Here's how the part is built. I have some questions about the finished solid (model axes, mm). A direction names the side the tool comes from. Coordinates: 2 decimals unless noted, no trailing zeros. Order: outer loops, then holes, each group sorted by start corner. A loop starts at its lowest first (then second) coordinate and runs counter-clockwise, first axis right, second up. Notation, with made-up numbers: M 87,-11.75 L 145,-11.75 A19 cw 145,-1.75 Z; hole C 70.25,70.25 d2. An arc over 180 degrees is marked long. Answer as CSV lines item,"result". Start each with the question number.
Autodesk Inventor part; units mm, degrees
ref_plane "YZ Plane" through (0, 0, 0) normal (1, 0, 0) x (0, 1, 0)
ref_plane "XZ Plane" through (0, 0, 0) normal (0, 1, 0) x (-1, 0, 0)
ref_plane "XY Plane" through (0, 0, 0) normal (0, 0, 1) x (1, 0, 0)
sketch "Esquisse1" plane through (0, 0, 0) normal (0, 1, 0) x (-1, 0, 0)
  line L0 (2.8537, 2.5756) -> (-12.1463, 2.5756)
  line L1 (-12.1463, 2.5756) -> (-12.1463, -7.4244)
  line L2 (-12.1463, -7.4244) -> (2.8537, -7.4244)
  line L3 (2.8537, -7.4244) -> (2.8537, 2.5756)
  point P0 (0, 0)
  dimension "d0" = 10
  dimension "d1" = 15
extrude "Extrusion1" add sketch "Esquisse1" along normal blind 3
sketch "Esquisse2" plane through (0, 3, 0) normal (0, 1, 0) x (1, 0, 0)
  line L0 (-2.8537, 7.4244) -> (-2.8537, -2.5756)
  line L1 (12.1463, 7.4244) -> (-2.8537, 7.4244)
  line L2 (-2.8537, -2.5756) -> (0.1463, -2.5756)
  line L3 (0.1463, -2.5756) -> (0.1463, 7.4244)
  line L4 (0.1463, 7.4244) -> (-2.8537, 7.4244)
  line L5 (-2.8537, 7.4244) -> (-2.8537, -2.5756)
  point P0 (0, 0)
  dimension "d4" = 3
extrude "Extrusion2" add sketch "Esquisse2" along normal blind 40
sketch "Esquisse3" plane through (0, 3, 0) normal (0, 1, 0) x (1, 0, 0)
  circle A0 centre (3.1463, 2.4244) radius 1.5
  circle A1 centre (9.1463, 2.4244) radius 1.5
  line L0 (12.1463, -2.5756) -> (12.1463, 7.4244)
  line L1 (0.1463, -2.5756) -> (12.1463, -2.5756)
  line L2 (0.1463, -2.5756) -> (0.1463, 7.4244)
  point P0 (0, 0)
  dimension "d7" = 3
  dimension "d8" = 3
  dimension "d9" = 3
  dimension "d10" = 5
  dimension "d11" = 5
  dimension "d12" = 3
extrude "Extrusion3" cut sketch "Esquisse3" against normal through all
sketch "Esquisse4" plane through (0, 3, 0) normal (0, 1, 0) x (1, 0, 0)
  line L0 (0.1463, -2.5756) -> (12.1463, -2.5756)
  line L1 (0.1463, -2.5756) -> (5.1463, -2.5756)
  line L2 (5.1463, -2.5756) -> (5.1463, -1.5756)
  line L3 (5.1463, -1.5756) -> (0.1463, -1.5756)
  line L4 (0.1463, -1.5756) -> (0.1463, -2.5756)
  line L5 (12.1463, 7.4244) -> (0.1463, 7.4244)
  line L6 (0.1463, 7.4244) -> (5.1463, 7.4244)
  line L7 (5.1463, 7.4244) -> (5.1463, 6.4244)
  line L8 (5.1463, 6.4244) -> (0.1463, 6.4244)
  line L9 (0.1463, 6.4244) -> (0.1463, 7.4244)
  point P0 (0, 0)
  dimension "d15" = 1
  dimension "d16" = 1
  dimension "d17" = 5
extrude "Extrusion4" add sketch "Esquisse4" along normal blind 5
chamfer "Chanfrein1" distance 5 angle 45 1 edges at (5.1463, 8, 2.0756)
chamfer "Chanfrein2" distance 5 angle 45 1 edges at (5.1463, 8, -6.9244)
sketch "Esquisse5" plane through (0.1463, 43, 2.5756) normal (1, 0, 0) x (0, 0, -1)
  circle A0 centre (5, -3) radius 1.5
  line L0 (0, -35) -> (0, 0)
  line L1 (0, 0) -> (10, 0)
  point P0 (2.5756, -43)
  dimension "d26" = 3
  dimension "d27" = 5
  dimension "d28" = 3
extrude "Extrusion5" cut sketch "Esquisse5" against normal through all
properties part number "equerre-bras"
1) Suppose I cut it at B-B on z = -2. Please give me the cut outline in (x, y) (3 decimals).
2) Suppose I cut it at A-A on y = 40. Please give me the cut outline in (x, z), plus the area to 3 significant figures.
3) I need wall thicknesses on line 1 (X direction, y = 36, z = 0); line 2 (Y direction, x = 3.75, z = -5); line 3 (Y direction, x = -2, z = -3). Which ranges of each line are inside material? Lowest first, please. Write a range as [from, to].
4) Which directions (+Z, -Z, +X, -X, +Y, -Y) give clear straight access to the entire face, cutting with the end or side of a thin tool? Please do faces 4 (the face through (-1, 43, -2)), 5 (the face through (2, 5, 1.576)).
5) Suppose I cut it at C-C on x = -1.75. Please give me the cut outline in (y, z), plus the area to 3 significant figures.
6) If we mould it in two halves opening along X, with no side actions, what happens to faces 1 (the face through (-1.333, 38.536, -2.099)), 2 (the face through (12.146, 1, -2)), 3 (the face through (3.95, 1.52, -3.69))? For each: released by +X, released by -X, zero draft, split by the parting line, or undercut.
7) Will these pins go through, and if not, where does the flat tip stop? pin 1 Ø3 at (x, z) = (6.5, -4) entering from +Y; pin 2 Ø5 at (y, z) = (40, -2.42) entering from +X; pin 3 Ø8 at (x, y) = (8, 9) entering from +Z.
8) Suppose I cut it at D-D on x = 3.5. Please give me the cut outline in (y, z), plus the area to 3 significant figures.
Output:
1,outline,"M -2.854,0 L 1.708,0 L 1.708,3 L 0.146,3 L 0.146,38.561 L -2.854,38.561 Z; M -2.854,41.439 L 0.146,41.439 L 0.146,43 L -2.854,43 Z; M 4.585,0 L 7.708,0 L 7.708,3 L 4.585,3 Z; M 10.585,0 L 12.146,0 L 12.146,3 L 10.585,3 Z"
2,outline,"M -2.85,-7.42 L 0.15,-7.42 L 0.15,-3.92 L -2.85,-3.92 Z; M -2.85,-0.92 L 0.15,-0.92 L 0.15,2.58 L -2.85,2.58 Z"
2,area,"21.0 mm²"
3,line 1,"[-2.85, 0.15]"
3,line 2,"[0, 3]"
3,line 3,"[0, 38.61], [41.39, 43]"
4,face 4,"+Z, -Z, +X, -X, +Y"
4,face 5,"+X, +Y"
5,outline,"M 0,-7.42 L 43,-7.42 L 43,2.58 L 0,2.58 Z; hole C 40,-2.42 d3"
5,area,"423 mm²"
6,face 1,"zero draft"
6,face 2,"released by +X"
6,face 3,"undercut"
7,pin 1,"y = 3"
7,pin 2,"x = 0.15"
7,pin 3,"through"
8,outline,"M 0,-7.42 L 4.65,-7.42 L 4.65,-6.42 L 3,-6.42 L 3,-3.88 L 0,-3.88 Z; M 0,-0.97 L 3,-0.97 L 3,1.58 L 4.65,1.58 L 4.65,2.58 L 0,2.58 Z"
8,area,"24.5 mm²"
